Read the model definition and answer for the solid it produces. Units are mm, in the model's axes. Face numbers are marked on the shaded views. Coordinates: 2 decimals unless noted, no trailing zeros. Order: outer loops, then holes, each group sorted by start corner. A loop starts at its lowest first (then second) coordinate and runs counter-clockwise, first axis right, second up.
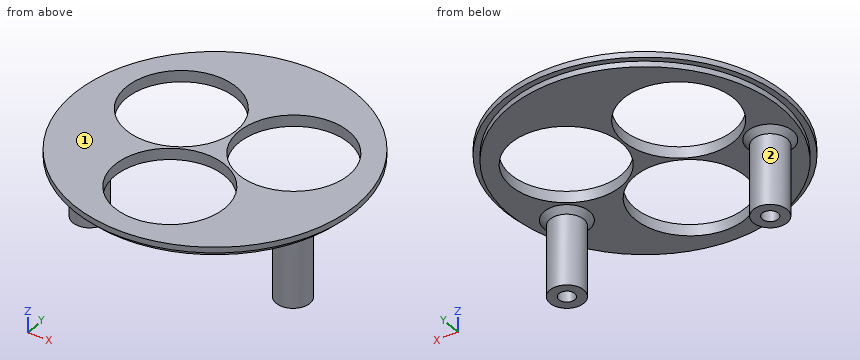
Autodesk Inventor part; units mm, degrees
ref_plane "YZ Plane" through (0, 0, 0) normal (1, 0, 0) x (0, 1, 0)
ref_plane "XZ Plane" through (0, 0, 0) normal (0, 1, 0) x (-1, 0, 0)
ref_plane "XY Plane" through (0, 0, 0) normal (0, 0, 1) x (1, 0, 0)
sketch "Sketch1" plane through (0, 0, 0) normal (0, 0, 1) x (1, 0, 0)
  circle A0 centre (-9.959, 5.75) radius 9.75
  circle A1 centre (0, -11.5) radius 9.75
  circle A2 centre (9.959, 5.75) radius 9.75
  circle A3 centre (0, 0) radius 25
  circle A4 centre (-18, -6) radius 1.4
  circle A5 centre (18, -6) radius 1.4
  circle A6 centre (18, -6) radius 3
  circle A7 centre (-18, -6) radius 3
  circle A8 centre (0, 0) radius 24
  dimension "d0" = 19.918
  dimension "d1" = 5.75
  dimension "d3" = 19.5
  dimension "d4" = 9.959
  dimension "d5" = 17.25
  dimension "d6" = 50
  dimension "d9" = 18
  dimension "d10" = 18
  dimension "d11" = 6
  dimension "d12" = 2.8
  dimension "d13" = 6
  dimension "d20" = 1
extrude "Extrusion1" add sketch "Sketch1" along normal blind 2 contours A3 | A4 | A5 | A6 | A7 | A8
extrude "Extrusion2" add sketch "Sketch1" against normal blind 13.5 contours A6 | A7
chamfer "Chamfer1" distance 1 angle 45 2 edges at (15, -6, 0) (-21, -6, 0)
extrude "Extrusion3" cut sketch "Sketch1" along normal blind 1 contours A3
properties part number "Housing_Front"
1) A cutting plane is placed at B-B, the plane y = 5.75. Determine the outline of the cut face in (x, z).
A:
outline: (-24.33, 1) - (-23.3, 1) - (-23.3, 0) - (-19.71, 0) - (-19.71, 2) - (-24.33, 2) - close; (-0.21, 0) - (0.21, 0) - (0.21, 2) - (-0.21, 2) - close; (19.71, 0) - (23.3, 0) - (23.3, 1) - (24.33, 1) - (24.33, 2) - (19.71, 2) - close
2) Flat-ended cylindrical pins translate along their axes: pin 1 Ø4 at (x, y) = (13.5, 15) entering from -Z; pin 2 Ø8 at (y, z) = (11, -3.5) entering from +X; pin 3 Ø2 at (y, z) = (-7, -5.5) entering from +X. Find the tip coordinate at first contact, or state that the pin passes through.
A:
pin 1: stops at z = 0
pin 2: stops at x = 22.22
pin 3: stops at x = 21
3) A cutting plane is placed at C-C, the plane x = 7. Determine the outline of the cut face in (y, z).
A:
outline: (-24, 1) - (-22.96, 1) - (-22.96, 0) - (-18.29, 0) - (-18.29, 2) - (-24, 2) - close; (-4.71, 0) - (-3.54, 0) - (-3.54, 2) - (-4.71, 2) - close; (15.04, 0) - (22.96, 0) - (22.96, 1) - (24, 1) - (24, 2) - (15.04, 2) - close
4) A cutting plane is placed at A-A, the plane z = -2.75. Determine the outline of the cut face in (x, y), and give its area (3 significant figures).
A:
outline: circle Ø6 at (-18, -6); circle Ø6 at (18, -6); hole circle Ø2.8 at (-18, -6); hole circle Ø2.8 at (18, -6)
area: 44.2 mm2
5) A cutting plane is placed at D-D, the plane y = -20. Determine the outline of the cut face in (x, z).
A:
outline: (-15, 1) - (-13.27, 1) - (-13.27, 0) - (-4.78, 0) - (-4.78, 2) - (-15, 2) - close; (4.78, 0) - (13.27, 0) - (13.27, 1) - (15, 1) - (15, 2) - (4.78, 2) - close
6) Determine the mould class of the marked faces 1 and 2 for opening direction X: pulls with the +X half, pulls with the -X half, needs draft (parallel to the pull), parting line crosses it, or undercut.
A:
face 1: needs draft
face 2: undercut
7) Straight lines are drawn through the part: line 1 (Y direction, x = -18, z = -1.5); line 2 (Y direction, x = 0, z = 1.25); line 3 (X direction, y = 8.5, z = 0.75). For each, find the intervals that lie inside material, in ascending order.
A:
line 1: y = -9 to -7.4, -4.6 to -3
line 2: y = -25 to -21.25, -1.75 to 25
line 3: x = -22.44 to -19.31, -0.6 to 0.6, 19.31 to 22.44
